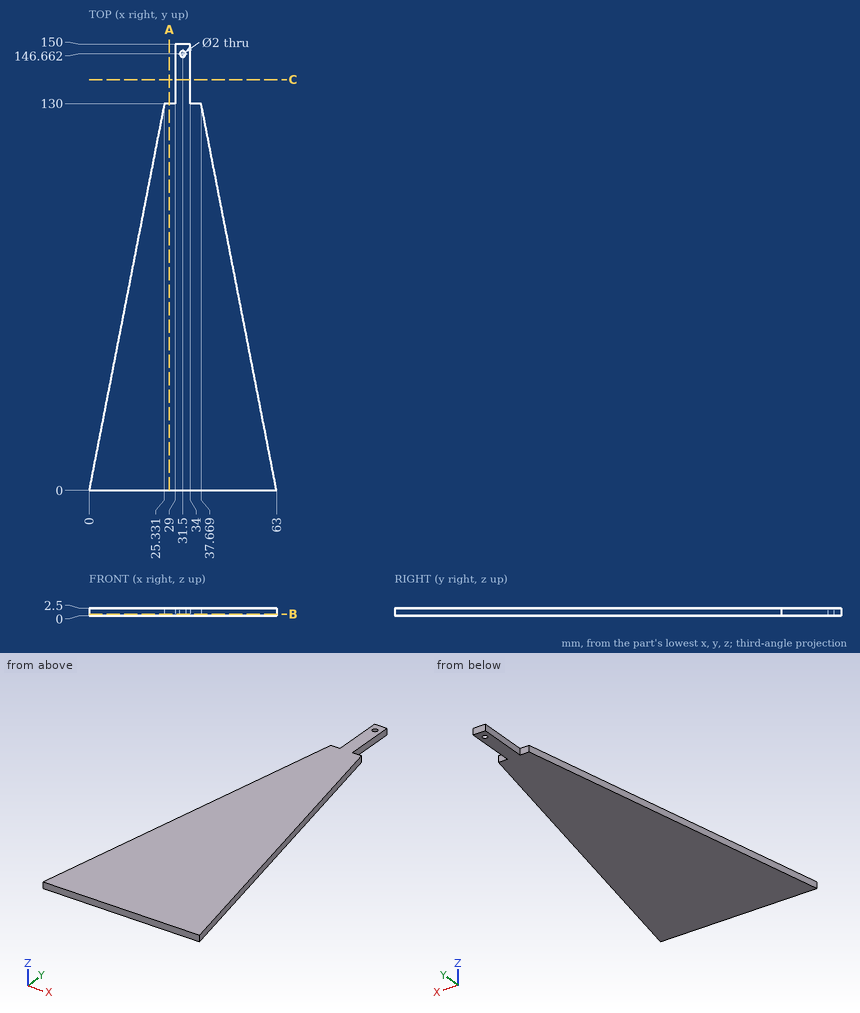
Answer from the drawing. Dimensions are ordinates in mm from the lowest x, y and z of the part. Round coordinates to 2 decimals unless told otherwise and drop trailing zeros. Write each loop counter-clockwise with the first axis right and the second up, starting at its lowest first coordinate (ties: lowest second). Pieces come first, ordered by that corner, then holes. Notation, with made-up numbers: M 46.25,-36.5 L 70.25,-36.5 A13 ccw 70.25,-20.5 Z; hole C 26,20 d6. An arc over 180 degrees is marked long. Write each question's results on one line, items separated by ' | '. Start each with the question number.
Item 1: Find section A-A on x = 27. Write down the section's boundary in (y, z).
Item 2: Straight lines are drawn through the part: probe 1 along Y at (x, z) = (31.5, 1.4); probe 2 along X at (y, z) = (138, 0.8); probe 3 along Y at (x, z) = (25.5, 1.85). For each, find the intervals that lie inside material, in ascending order.
Item 3: Find section B-B on z = 0.6. Write down the section's boundary in (x, y).
Item 4: Given pin 1 Ø3 at (x, y) = (19.5, 116) entering from +Z; pin 2 Ø0.8 at (y, z) = (144.5, 2) entering from +X; pin 3 Ø8 at (x, y) = (14, 80) entering from -Z; pin 4 Ø1.2 at (y, z) = (138.5, 0.5) entering from -X, each flat-ended and moving along its own axis, determine where each tip first touches the part or whether it passes through.
Item 5: Find section C-C on y = 138. Write down the section's boundary in (x, z).
Answer block:
1) outline: M 0,0 L 130,0 L 130,2.5 L 0,2.5 Z
2) probe 1: y = 0 to 145.66, 147.66 to 150 | probe 2: x = 29 to 34 | probe 3: y = 0 to 130
3) outline: M 0,0 L 63,0 L 37.67,130 L 34,130 L 34,150 L 29,150 L 29,130 L 25.33,130 Z; hole C 31.5,146.66 d2
4) pin 1: passes through | pin 2: stops at x = 34 | pin 3: stops at z = 0 | pin 4: stops at x = 29
5) outline: M 29,0 L 34,0 L 34,2.5 L 29,2.5 Z
